The listing builds one solid part. Answer for the finished solid, in the listing's coordinates (mm). Give positions to 0.01 mm unless a question says otherwise; leave off trailing zeros. Write each loop counter-clockwise with the first axis right and the second up, starting at its lowest first coordinate (ties: lowest second). Pieces come first, ordered by that corner, then holes. Notation, with made-up numbers: M 72,24.5 L 108,24.5 A32 cw 108,55.5 Z; hole C 61,74 d4. An arc over 180 degrees is marked long. Return JSON: item names as keys, results as strings.
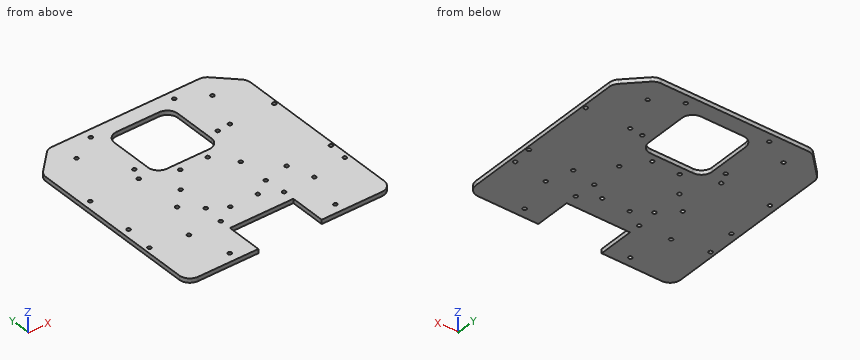
from build123d import *

# Parameters (mm, degrees)
EXTRUDE_1_DEPTH      = 4
SKETCH_6_R           = 1.75
CUT_EXTRUDE_3_DEPTH  = 4
SKETCH_4_R           = 1.75
CUT_EXTRUDE_4_DEPTH  = 4
SKETCH_7_R           = 1.75
CUT_EXTRUDE_5_DEPTH  = 4
SKETCH_8_R           = 1.75
CUT_EXTRUDE_6_DEPTH  = 4
CUT_EXTRUDE_7_DEPTH  = 4
SKETCH_10_R          = 1.75
SKETCH_10_R_2        = 1.749999998
CUT_EXTRUDE_9_DEPTH  = 4
CUT_EXTRUDE_10_REACH = 358.759
SKETCH_11_R          = 1.75
SKETCH_12_R          = 1.75
CUT_EXTRUDE_13_DEPTH = 357.758930869
SKETCH_13_W          = 60
SKETCH_13_H          = 33.978821531
CUT_EXTRUDE_14_DEPTH = 10
SKETCH_14_W          = 60
SKETCH_14_H          = 10
CUT_EXTRUDE_16_DEPTH = 10


with BuildPart() as part:
    # 草图3 → 凸台-拉伸1 (new body)
    with BuildSketch(Plane.XY):
        with BuildLine():
            Line((73.505746565, 259.089488009), (196.937204075, 259.089488009))
            ThreePointArc((196.937204075, 259.089488009), (204.590872722, 257.56707866), (211.079339699, 253.231623633))
            Line((211.079339699, 253.231623633), (239.363610944, 224.947352388))
            ThreePointArc((239.363610944, 224.947352388), (243.69906597, 218.458885412), (245.22147532, 210.805216764))
            Line((245.22147532, 210.805216764), (245.22147532, 54.089488009))
            ThreePointArc((245.22147532, 54.089488009), (239.363610944, 39.947352386), (225.22147532, 34.089488009))
            Line((225.22147532, 34.089488009), (45.221475318, 34.089488009))
            ThreePointArc((45.221475318, 34.089488009), (31.079339694, 39.947352386), (25.221475318, 54.089488009))
            Line((25.221475318, 54.089488009), (25.221475318, 210.805216762))
            ThreePointArc((25.221475318, 210.805216762), (26.743884667, 218.458885409), (31.079339694, 224.947352386))
            Line((31.079339694, 224.947352386), (59.363610941, 253.231623633))
            ThreePointArc((59.363610941, 253.231623633), (65.852077918, 257.56707866), (73.505746565, 259.089488009))
        make_face()
    extrude(amount=EXTRUDE_1_DEPTH)

    # 草图6 → 切除-拉伸3 (cut)
    with BuildSketch(Plane.XY.offset(4)):
        with Locations((187.22147532, 181.880072532)):
            Circle(SKETCH_6_R)
        with Locations((229.22147532, 181.880072532)):
            Circle(SKETCH_6_R)
        with Locations((229.22147532, 113.880072532)):
            Circle(SKETCH_6_R)
        with Locations((187.22147532, 113.880072532)):
            Circle(SKETCH_6_R)
    extrude(amount=-CUT_EXTRUDE_3_DEPTH, mode=Mode.SUBTRACT)

    # 草图4 → 切除-拉伸4 (cut)
    with BuildSketch(Plane.XY.offset(4)):
        with Locations((174.691475319, 232.74535793)):
            Circle(SKETCH_4_R)
        with Locations(Location((174.691475319, 180.63535793, 0), (0, 0, 180))):
            Circle(SKETCH_4_R)
        with Locations((95.751475319, 180.63535793)):
            Circle(SKETCH_4_R)
        with Locations(Location((95.751475319, 232.74535793, 0), (0, 0, 180))):
            Circle(SKETCH_4_R)
        with Locations((165.22147532, 89.06830954)):
            Circle(SKETCH_4_R)
        with Locations(Location((105.22147532, 89.06830954, 0), (0, 0, 180))):
            Circle(SKETCH_4_R)
    extrude(amount=-CUT_EXTRUDE_4_DEPTH, mode=Mode.SUBTRACT)

    # 草图7 → 切除-拉伸5 (cut)
    with BuildSketch(Plane.XY.offset(4)):
        with Locations((122.221475319, 159.089488009)):
            Circle(SKETCH_7_R)
        with Locations((148.221475319, 159.089488009)):
            Circle(SKETCH_7_R)
        with Locations((122.221475319, 99.089488009)):
            Circle(SKETCH_7_R)
        with Locations((148.221475319, 99.089488009)):
            Circle(SKETCH_7_R)
    extrude(amount=-CUT_EXTRUDE_5_DEPTH, mode=Mode.SUBTRACT)

    # 草图8 → 切除-拉伸6 (cut)
    with BuildSketch(Plane.XY.offset(4)):
        with Locations((227.720064334, 95.494716411)):
            Circle(SKETCH_8_R)
        with Locations((185.293657462, 53.06830954)):
            Circle(SKETCH_8_R)
        with Locations(Location((42.722886307, 95.494716411, 0), (0, 0, 180))):
            Circle(SKETCH_8_R)
        with Locations(Location((85.149293178, 53.06830954, 0), (0, 0, 180))):
            Circle(SKETCH_8_R)
    extrude(amount=-CUT_EXTRUDE_6_DEPTH, mode=Mode.SUBTRACT)

    # 草图9 → 切除-拉伸7 (cut)
    with BuildSketch(Plane.XY.offset(4)):
        with BuildLine():
            Line((115.22147532, 166.324698125), (155.22147532, 166.324698125))
            ThreePointArc((155.22147532, 166.324698125), (162.292543132, 169.253630313), (165.22147532, 176.324698125))
            Line((165.22147532, 176.324698125), (165.22147532, 216.324698125))
            ThreePointArc((165.22147532, 216.324698125), (162.292543132, 223.395765937), (155.22147532, 226.324698125))
            Line((155.22147532, 226.324698125), (135.22147532, 226.324698125))
            Line((135.22147532, 226.324698125), (115.22147532, 226.324698125))
            ThreePointArc((115.22147532, 226.324698125), (108.150407508, 223.395765937), (105.22147532, 216.324698125))
            Line((105.22147532, 216.324698125), (105.22147532, 196.104283633))
            Line((105.22147532, 196.104283633), (105.22147532, 176.324698125))
            ThreePointArc((105.22147532, 176.324698125), (108.150407508, 169.253630313), (115.22147532, 166.324698125))
        make_face()
    extrude(amount=-CUT_EXTRUDE_7_DEPTH, mode=Mode.SUBTRACT)

    # 草图10 → 切除-拉伸9 (cut)
    with BuildSketch(Plane.XY.offset(4)):
        with Locations((106.721475319, 109.089488009)):
            Circle(SKETCH_10_R)
        with Locations((163.721475321, 109.089488009)):
            Circle(SKETCH_10_R_2)
        with Locations((106.721475319, 139.089488009)):
            Circle(SKETCH_10_R)
        with Locations(Location((163.721475321, 139.089488009, 0), (0, 0, 180))):
            Circle(SKETCH_10_R)
    extrude(amount=-CUT_EXTRUDE_9_DEPTH, mode=Mode.SUBTRACT)

    # 草图11 → 切除-拉伸10 (cut, up to next)
    with BuildSketch(Plane.XY.offset(4), mode=Mode.PRIVATE) as cut_extrude_10_sk1:
        with Locations((70.852077918, 218.458885409)):
            Circle(SKETCH_11_R)
    cut_extrude_10_tool1 = extrude(cut_extrude_10_sk1.sketch, amount=-CUT_EXTRUDE_10_REACH, mode=Mode.PRIVATE) & part.part
    # 草图11 → 切除-拉伸10 (cut, up to next)
    with BuildSketch(Plane.XY.offset(4), mode=Mode.PRIVATE) as cut_extrude_10_sk2:
        with Locations((75.852077918, 90.084611013)):
            Circle(SKETCH_11_R)
    cut_extrude_10_tool2 = extrude(cut_extrude_10_sk2.sketch, amount=-CUT_EXTRUDE_10_REACH, mode=Mode.PRIVATE) & part.part
    # 草图11 → 切除-拉伸10 (cut, up to next)
    with BuildSketch(Plane.XY.offset(4), mode=Mode.PRIVATE) as cut_extrude_10_sk3:
        with Locations((194.590872722, 90.084611013)):
            Circle(SKETCH_11_R)
    cut_extrude_10_tool3 = extrude(cut_extrude_10_sk3.sketch, amount=-CUT_EXTRUDE_10_REACH, mode=Mode.PRIVATE) & part.part
    # 草图11 → 切除-拉伸10 (cut, up to next)
    with BuildSketch(Plane.XY.offset(4), mode=Mode.PRIVATE) as cut_extrude_10_sk4:
        with Locations((199.590872722, 218.458885409)):
            Circle(SKETCH_11_R)
    cut_extrude_10_tool4 = extrude(cut_extrude_10_sk4.sketch, amount=-CUT_EXTRUDE_10_REACH, mode=Mode.PRIVATE) & part.part
    add(cut_extrude_10_tool1.solids().sort_by_distance((70.852078, 218.458885, 4))[0], mode=Mode.SUBTRACT)
    add(cut_extrude_10_tool2.solids().sort_by_distance((75.852078, 90.084611, 4))[0], mode=Mode.SUBTRACT)
    add(cut_extrude_10_tool3.solids().sort_by_distance((194.590873, 90.084611, 4))[0], mode=Mode.SUBTRACT)
    add(cut_extrude_10_tool4.solids().sort_by_distance((199.590873, 218.458885, 4))[0], mode=Mode.SUBTRACT)

    # 草图12 → 切除-拉伸13 (cut, through all)
    with BuildSketch(Plane.XY.offset(4)):
        with Locations((90.961423691, 169.312171827)):
            Circle(SKETCH_12_R)
        with Locations((90.961423691, 123.312171827)):
            Circle(SKETCH_12_R)
        with Locations((44.961423691, 123.312171827)):
            Circle(SKETCH_12_R)
        with Locations((44.961423691, 169.312171827)):
            Circle(SKETCH_12_R)
    extrude(amount=-CUT_EXTRUDE_13_DEPTH, mode=Mode.SUBTRACT)

    # 草图13 → 切除-拉伸14 (cut)
    with BuildSketch(Plane.XY.offset(4)):
        with Locations((135.22147532, 51.078898775)):
            Rectangle(SKETCH_13_W, SKETCH_13_H)
    extrude(amount=-CUT_EXTRUDE_14_DEPTH, mode=Mode.SUBTRACT)

    # 草图14 → 切除-拉伸16 (cut)
    with BuildSketch(Plane.XY):
        with BuildLine():
            Line((38.221475318, 210.805216762), (38.221475318, 213.805216762))
            ThreePointArc((38.221475318, 213.805216762), (38.982679993, 217.632051085), (41.150407506, 220.876284574))
            Line((41.150407506, 220.876284574), (58.434678753, 238.160555821))
            ThreePointArc((58.434678753, 238.160555821), (61.678912242, 240.328283334), (65.505746565, 241.089488009))
            Line((65.505746565, 241.089488009), (73.505746565, 241.089488009))
            Line((73.505746565, 241.089488009), (196.937204075, 241.089488009))
            Line((196.937204075, 241.089488009), (204.937204075, 241.089488009))
            ThreePointArc((204.937204075, 241.089488009), (208.764038399, 240.328283334), (212.008271887, 238.160555821))
            Line((212.008271887, 238.160555821), (229.292543132, 220.876284576))
            ThreePointArc((229.292543132, 220.876284576), (231.460270645, 217.632051088), (232.22147532, 213.805216764))
            Line((232.22147532, 213.805216764), (232.22147532, 54.089488009))
            ThreePointArc((232.22147532, 54.089488009), (229.292543132, 47.018420197), (222.22147532, 44.089488009))
            Line((222.22147532, 44.089488009), (175.22147532, 44.089488009))
            Line((175.22147532, 44.089488009), (165.22147532, 44.089488009))
            Line((165.22147532, 44.089488009), (165.22147532, 34.089488009))
            Line((165.22147532, 34.089488009), (225.22147532, 34.089488009))
            ThreePointArc((225.22147532, 34.089488009), (239.363610944, 39.947352386), (245.22147532, 54.089488009))
            Line((245.22147532, 54.089488009), (245.22147532, 210.805216764))
            ThreePointArc((245.22147532, 210.805216764), (243.69906597, 218.458885412), (239.363610944, 224.947352388))
            Line((239.363610944, 224.947352388), (211.079339699, 253.231623633))
            ThreePointArc((211.079339699, 253.231623633), (204.590872722, 257.56707866), (196.937204075, 259.089488009))
            Line((196.937204075, 259.089488009), (73.505746565, 259.089488009))
            ThreePointArc((73.505746565, 259.089488009), (65.852077918, 257.56707866), (59.363610941, 253.231623633))
            Line((59.363610941, 253.231623633), (31.079339694, 224.947352386))
            ThreePointArc((31.079339694, 224.947352386), (26.743884667, 218.458885409), (25.221475318, 210.805216762))
            Line((25.221475318, 210.805216762), (25.221475318, 54.089488009))
            ThreePointArc((25.221475318, 54.089488009), (31.079339694, 39.947352386), (45.221475318, 34.089488009))
            Line((45.221475318, 34.089488009), (105.22147532, 34.089488009))
            Line((105.22147532, 34.089488009), (105.22147532, 44.089488009))
            Line((105.22147532, 44.089488009), (95.22147532, 44.089488009))
            Line((95.22147532, 44.089488009), (48.221475318, 44.089488009))
            ThreePointArc((48.221475318, 44.089488009), (41.150407506, 47.018420197), (38.221475318, 54.089488009))
            Line((38.221475318, 54.089488009), (38.221475318, 210.805216762))
        make_face()
        with Locations((135.22147532, 73.06830954)):
            Rectangle(SKETCH_14_W, SKETCH_14_H)
    extrude(amount=CUT_EXTRUDE_16_DEPTH, mode=Mode.SUBTRACT)


solid = part.part
Item 1: A cutting plane is placed at A-A, the plane y = 189.5. Write down the section's boundary in (x, z).
Geometry results:
{"outline": "M 38.22,0 L 105.22,0 L 105.22,4 L 38.22,4 Z; M 165.22,0 L 232.22,0 L 232.22,4 L 165.22,4 Z"}
Item 2: Find the intervals of material crossed by line 1 (X direction, y = 218.5, z = 2.25); line 2 (Y direction, x = 141, z = 2.85); line 3 (Y direction, x = 186.5, z = 1.2), in increasing order.
Geometry results:
{"line 1": "x = 39.39 to 69.1, 72.6 to 105.46, 164.98 to 197.84, 201.34 to 231.05", "line 2": "y = 78.07 to 166.32, 226.32 to 241.09", "line 3": "y = 44.09 to 51.8, 54.34 to 112.29, 115.47 to 180.29, 183.47 to 241.09"}
Item 3: Given pin 1 Ø3 at (x, y) = (148.22, 159.09) entering from -Z, flat-ended and moving along its own axis, determine where the tip first touches the part or whether it passes through.
Geometry results:
{"pin 1": "passes through"}
Item 4: A cutting plane is placed at B-B, the plane z = 1.65. Count the separate pieces of the cut face and the enclosed holes in it, plus the area to 3 significant figures.
Geometry results:
{"separate pieces": "1", "enclosed holes": "31", "area": "31,800 mm2"}
